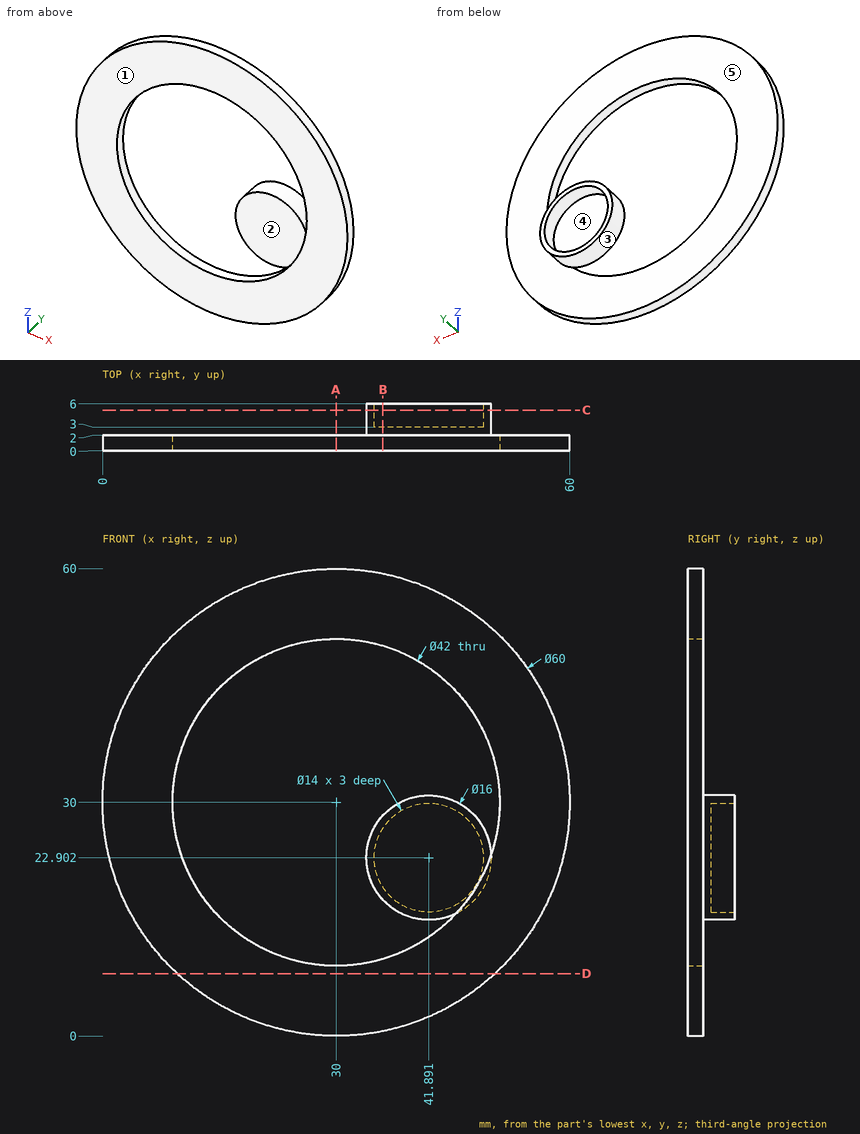
Geometry: see drawing. Coordinates: mm, zero at the bounding-box minimum. A direction names the side the tool comes from. Coordinates: 2 decimals unless noted, no trailing zeros. Loops run counter-clockwise (first coordinate to the right, second up) from the corner with the lowest first, then second, coordinate; pieces in that order, holes last. Notation, with made-up numbers: M -18,72.25 L -13,72.25 A22 cw -13,100.25 Z; hole C 10,58 d2. An arc over 180 degrees is marked long. Answer in a Markdown table with one row per item.
1. Material intervals for line 1 (Z direction, x = 30, y = 1.65); line 2 (Y direction, x = 22, z = 5.5), sorted ascending.
Response:
| item | result |
|---|---|
| line 1 | z = 0 to 9, 51 to 60 |
| line 2 | y = 0 to 2 |
2. Draft query along Z for the marked faces 3, 4 and 5. Return one class per face: pulls with the +Z half, pulls with the -Z half, needs draft (parallel to the pull), parting line crosses it, or undercut.
Response:
| item | result |
|---|---|
| face 3 | parting line crosses it |
| face 4 | undercut |
| face 5 | needs draft |
3. Section D-D, the plane z = 8. Output: boundary loops of the cut face in (x, y).
Response:
| item | result |
|---|---|
| outline | M 9.6,0 L 50.4,0 L 50.4,2 L 9.6,2 Z |
4. Section C-C, the plane y = 5.2. Output: boundary loops of the cut face in (x, z).
Response:
| item | result |
|---|---|
| outline | C 41.89,22.9 d16; hole C 41.89,22.9 d14 |
5. Section B-B, the plane x = 36. Output: boundary loops of the cut face in (y, z) (1 decimal).
Response:
| item | result |
|---|---|
| outline | M 0,0.6 L 2,0.6 L 2,9.9 L 0,9.9 Z; M 0,50.1 L 2,50.1 L 2,59.4 L 0,59.4 Z; M 2,17.5 L 6,17.5 L 6,19.1 L 3,19.1 L 3,26.7 L 6,26.7 L 6,28.3 L 2,28.3 Z |
6. Section A-A, the plane x = 30. Output: boundary loops of the cut face in (y, z).
Response:
| item | result |
|---|---|
| outline | M 0,0 L 2,0 L 2,9 L 0,9 Z; M 0,51 L 2,51 L 2,60 L 0,60 Z |
7. Reachability of the marked faces 1 and 2 from +Z, -Z, +X, -X, +Y, -Y: full face, straight path, thin tool, end or side. Return the list, or none.
Response:
| item | result |
|---|---|
| face 1 | +Z, -Z, +X, -X, -Y |
| face 2 | -Y |
8. First-contact query: pin 1 (8 mm diameter, centred on x = 54, z = 19.5, fed in from +Y); pin 2 (12.5 mm diameter, centred on x = 41.89, z = 22.9, fed in from -Y); pin 3 (7 mm diameter, centred on x = 40.5, z = 23, fed in from +Y). Flat tips, straight axial feed; report the tip coordinate or a pass-through.
Response:
| item | result |
|---|---|
| pin 1 | stops at y = 2 |
| pin 2 | stops at y = 2 |
| pin 3 | stops at y = 3 |
